Work out the finished part from the listing and answer in its coordinate system (mm). A direction names the side the tool comes from. Give positions to 0.01 mm unless a question says otherwise; leave off trailing zeros. Loops run counter-clockwise (first coordinate to the right, second up) from the corner with the lowest first, then second, coordinate; pieces in that order, holes last. Notation, with made-up numbers: (61, 41) - (99, 41) arc R11 cw to (99, 45) - close; hole circle Ø2 at (62, -8.75). An arc over 180 degrees is marked (long way). One line per item, written item: value.
Autodesk Inventor part; units mm, degrees
ref_plane "YZ Plane" through (0, 0, 0) normal (1, 0, 0) x (0, 1, 0)
ref_plane "XZ Plane" through (0, 0, 0) normal (0, 1, 0) x (-1, 0, 0)
ref_plane "XY Plane" through (0, 0, 0) normal (0, 0, 1) x (1, 0, 0)
sketch "スケッチ1" plane through (0, 0, 0) normal (0, 0, 1) x (1, 0, 0)
  line L0 (0, 0) -> (20, 0)
  line L1 (20, 0) -> (20, 40)
  line L2 (20, 40) -> (0, 40)
  line L3 (0, 40) -> (0, 0)
  line L4 (2, 2) -> (18, 2)
  line L5 (18, 2) -> (18, 38)
  line L6 (18, 38) -> (2, 38)
  line L7 (2, 38) -> (2, 2)
  dimension "d0" = 20
  dimension "d1" = 40
  dimension "d2" = 2
extrude "押し出し1" add sketch "スケッチ1" along normal blind 55
sketch "スケッチ2" plane through (20, 0, 0) normal (1, 0, 0) x (0, 0, -1)
  line L0 (0, 0) -> (0, 40)
  point P0 (-20, 20)
  dimension "d5" = 20
hole "穴1" at (20, 20, 20) direction (-1, 0, 0) diameter 12 depth 2
sketch "スケッチ3" plane through (0, 0, 0) normal (-1, 0, 0) x (0, 0, 1)
  line L0 (0, 40) -> (0, 0)
  line L1 (0, 40) -> (55, 40)
  point P0 (20, 20)
  point P1 (20, 11)
  point P2 (20, 29)
  dimension "d13" = 20
  dimension "d14" = 20
  dimension "d15" = 9
  dimension "d16" = 9
hole "穴2" at (0, 20, 20) direction (1, 0, 0) diameter 12 depth 2
hole "穴3" at (0, 11, 20) at (0, 29, 20) direction (1, 0, 0) diameter 3.1 depth 2
sketch "スケッチ4" plane through (0, 40, 0) normal (0, 1, 0) x (1, 0, 0)
  line L0 (20, 0) -> (0, 0)
  point P0 (10, -7.5)
  point P1 (10, -47.5)
  dimension "d31" = 7.5
  dimension "d32" = 47.5
hole "穴4" at (10, 40, 7.5) at (10, 40, 47.5) direction (0, -1, 0) diameter 3.1 depth 2
sketch "スケッチ5" plane through (0, 0, 0) normal (-1, 0, 0) x (0, 0, 1)
  line L0 (0, 0) -> (55, 0)
  line L1 (25, 0) -> (55, 35)
  line L2 (55, 2) -> (55, 38)
  line L3 (55, 40) -> (55, 0)
  dimension "d40" = 30
  dimension "d41" = 35
extrude "押し出し2" cut sketch "スケッチ5" against normal blind 55
properties part number "SU22_SQP_20_40_EU_sn" material "アルミニウム 6061-AHC"
1. Section C-C (y = 20) is taken. Write down the section's boundary in (x, z), and give its area (3 significant figures).
Output:
outline: (0, 0) - (2, 0) - (2, 14) - (0, 14) - close; (0, 26) - (2, 26) - (2, 42.14) - (0, 42.14) - close; (18, 0) - (20, 0) - (20, 14) - (18, 14) - close; (18, 26) - (20, 26) - (20, 42.14) - (18, 42.14) - close
area: 121 mm²
2. For faces 1 (the flat face through (2, 24, 27)), 2 (the cylindrical face through (1.014, 11.594, 21.432)), 3 (the flat face through (0, 25, 27)), determine the directions among +Z, -Z, +X, -X, +Y, -Y from which every point of the face is accessible in a straight line to the end or side of a thin tool.
Output:
face 1: +Z, -Z
face 2: -X
face 3: +Z, -Z, -X, +Y, -Y
3. Find the intervals of material crossed by line 1 along Y through (x, z) = (1.55, 20); line 2 along X through (y, z) = (37, 37.5); line 3 along Y through (x, z) = (8.75, 13.5), in increasing order.
Output:
line 1: y = 0 to 9.45, 12.55 to 14, 26 to 27.45, 30.55 to 40
line 2: x = 0 to 2, 18 to 20
line 3: y = 0 to 2, 38 to 40
4. Section A-A (z = 20) is taken. Write down the section's boundary in (x, y), and give its area (3 significant figures).
Output:
outline: (0, 0) - (20, 0) - (20, 14) - (18, 14) - (18, 2) - (2, 2) - (2, 9.45) - (0, 9.45) - close; (0, 12.55) - (2, 12.55) - (2, 14) - (0, 14) - close; (0, 26) - (2, 26) - (2, 27.45) - (0, 27.45) - close; (0, 30.55) - (2, 30.55) - (2, 38) - (18, 38) - (18, 26) - (20, 26) - (20, 40) - (0, 40) - close
area: 164 mm²
5. Section B-B (x = 16.75) is taken. Write down the section's boundary in (y, z), and give its area (3 significant figures).
Output:
outline: (0, 0) - (2, 0) - (2, 26.71) - (0, 25) - close; (38, 0) - (40, 0) - (40, 55) - (38, 55) - close
area: 162 mm²
6. The mould has two halves that part along Y. Classify faces 4 (the cylindrical face through (1.01, 27.69, 20.83)), 5 (the flat face through (1.81, 14.83, 37.71)), 6 (the flat face through (10, 40, 27)), 7 (the cylindrical face through (11.513, 38.986, 7.164)): released by +Y, released by -Y, zero draft, split by the parting line, or undercut.
Output:
face 4: undercut
face 5: released by -Y
face 6: released by +Y
face 7: zero draft
7. Section D-D (z = 47.5) is taken. Write down the section's boundary in (x, y), and give its area (3 significant figures).
Output:
outline: (0, 26.25) - (2, 26.25) - (2, 38) - (8.45, 38) - (8.45, 40) - (0, 40) - close; (11.55, 38) - (18, 38) - (18, 26.25) - (20, 26.25) - (20, 40) - (11.55, 40) - close
area: 80.8 mm²
